Part model, mm, in its own coordinate system. A direction names the side the tool comes from. Give positions to 0.01 mm unless a question says otherwise; leave off trailing zeros. Write each loop counter-clockwise with the first axis right and the second up, starting at its lowest first coordinate (ties: lowest second). Pieces come first, ordered by that corner, then holes.
from build123d import *

# Parameters (mm, degrees)
SKETCH1_R           = 1
BOSS_EXTRUDE1_DEPTH = 15
SKETCH2_R           = 1
CUT_EXTRUDE1_DEPTH  = 105.560998943
FILLET1_R           = 0.35
SKETCH4_R           = 1
SKETCH4_R_2         = 0.75
BOSS_EXTRUDE2_DEPTH = 15


with BuildPart() as part:
    # Sketch1 → Boss-Extrude1 (new body)
    with BuildSketch(Plane.XY):
        with BuildLine():
            Line((-3.91822664, -0.5), (-11.924682731, -0.5))
            Line((-11.924682731, -0.5), (-11.924682731, -3.5))
            Line((-11.924682731, -3.5), (-5.417794754, -3.5))
            ThreePointArc((-5.417794754, -3.5), (-2.957602121, -5.731935947), (0.287025, -6.443610529))
            Line((0.287025, -6.443610529), (97.091971847, -2.131518769))
            ThreePointArc((97.091971847, -2.131518769), (97.728368045, -2.205906231), (98.308583108, -2.477722522))
            ThreePointArc((98.308583108, -2.477722522), (103, 0), (98.308583108, 2.477722522))
            ThreePointArc((98.308583108, 2.477722522), (97.728368045, 2.205906231), (97.091971847, 2.131518769))
            Line((97.091971847, 2.131518769), (0.287025, 6.443610529))
            ThreePointArc((0.287025, 6.443610529), (-1.950218056, 6.148101295), (-3.948733974, 5.1))
            Line((-3.948733974, 5.1), (-6.571238743, 5.1))
            Line((-6.571238743, 5.1), (-6.571238743, 3.5))
            Line((-6.571238743, 3.5), (-11.924682731, 3.5))
            Line((-11.924682731, 3.5), (-11.924682731, 0.5))
            Line((-11.924682731, 0.5), (-3.91822664, 0.5))
            ThreePointArc((-3.91822664, 0.5), (-3.242430239, 2.255913594), (-1.830983342, 3.5))
            Line((-1.830983342, 3.5), (1.830983342, 3.5))
            ThreePointArc((1.830983342, 3.5), (2.255913594, -3.242430239), (-3.91822664, -0.5))
        make_face()
        Polygon((88.963478068, 1.645749001), (94.011025285, 1.447599375), (91.58632649, -0.977099421), align=None, mode=Mode.SUBTRACT)
        with BuildLine():
            ThreePointArc((3.206155917, -5.012291316), (5.643134431, -1.88614257), (5.575683387, 2.077078421))
            Line((5.575683387, 2.077078421), (12.307755133, -4.654993325))
            Line((12.307755133, -4.654993325), (3.206155917, -5.012291316))
        make_face(mode=Mode.SUBTRACT)
        Polygon((29.468467153, -3.981321833), (13.440872209, -4.610510983), (21.769264256, 3.717881064), align=None, mode=Mode.SUBTRACT)
        Polygon((44.134225049, -3.405593798), (30.60158423, -3.93683949), (37.633527485, 3.095103765), align=None, mode=Mode.SUBTRACT)
        Polygon((56.667764123, -2.91356946), (45.267342125, -3.361111456), (51.191324122, 2.562870541), align=None, mode=Mode.SUBTRACT)
        Polygon((67.379082477, -2.493079343), (57.800881199, -2.869087118), (62.777985726, 2.108017409), align=None, mode=Mode.SUBTRACT)
        Polygon((76.533108343, -2.133723259), (68.512199553, -2.448597), (72.680090819, 1.719294266), align=None, mode=Mode.SUBTRACT)
        Polygon((84.356252684, -1.826613081), (77.666225419, -2.089240916), (81.142552969, 1.387086634), align=None, mode=Mode.SUBTRACT)
        Polygon((91.042009123, -1.564152904), (85.48936976, -1.782130738), (88.374678359, 1.10317786), align=None, mode=Mode.SUBTRACT)
        Polygon((96.755739716, -1.339851173), (92.175126199, -1.519670561), (94.555342652, 0.860545892), align=None, mode=Mode.SUBTRACT)
        with Locations((100, 0)):
            Circle(SKETCH1_R, mode=Mode.SUBTRACT)
        Polygon((21.224946889, 4.304934547), (12.8520725, -4.067939842), (3.794955626, 4.989177032), align=None, mode=Mode.SUBTRACT)
        Polygon((30.01278452, -3.39426835), (22.358063966, 4.260452205), (37.089210118, 3.682157248), align=None, mode=Mode.SUBTRACT)
        Polygon((44.678542416, -2.818540315), (38.222327195, 3.637674906), (50.647006755, 3.149924024), align=None, mode=Mode.SUBTRACT)
        Polygon((57.21208149, -2.326515977), (51.780123831, 3.105441681), (62.233668359, 2.695070892), align=None, mode=Mode.SUBTRACT)
        Polygon((67.923399844, -1.90602586), (63.366785435, 2.650588549), (72.135773452, 2.306347749), align=None, mode=Mode.SUBTRACT)
        Polygon((77.07742571, -1.546669776), (73.268890528, 2.261865406), (80.598235603, 1.974140117), align=None, mode=Mode.SUBTRACT)
        Polygon((84.900570051, -1.239559598), (81.731352679, 1.929657774), (87.830360992, 1.690231343), align=None, mode=Mode.SUBTRACT)
    extrude(amount=-BOSS_EXTRUDE1_DEPTH)

    # Sketch2 → Cut-Extrude1 (cut, through all)
    with BuildSketch(Plane(origin=(0, 3.5, 0), x_dir=(1, 0, 0), z_dir=(0, 1, 0))):
        with Locations(Location((-8.671238743, 11.25, 0), (0, 0, 270))):
            Circle(SKETCH2_R)
        with Locations(Location((-8.671238743, 3.75, 0), (0, 0, 270))):
            Circle(SKETCH2_R)
    extrude(amount=-CUT_EXTRUDE1_DEPTH, mode=Mode.SUBTRACT)

    # Fillet1
    fillet1_edges = [part.edges().sort_by_distance(p)[0] for p in [
        (92.175126199, -1.519670561, -7.5),
        (96.755739716, -1.339851173, -7.5),
        (94.555342652, 0.860545892, -7.5),
        (87.830360992, 1.690231343, -7.5),
        (81.731352679, 1.929657774, -7.5),
        (84.900570051, -1.239559598, -7.5),
        (88.963478068, 1.645749001, -7.5),
        (91.58632649, -0.977099421, -7.5),
        (94.011025285, 1.447599375, -7.5),
        (72.680090819, 1.719294266, -7.5),
        (68.512199553, -2.448597, -7.5),
        (76.533108343, -2.133723259, -7.5),
        (63.366785435, 2.650588549, -7.5),
        (67.923399844, -1.90602586, -7.5),
        (72.135773452, 2.306347749, -7.5),
        (57.800881199, -2.869087118, -7.5),
        (67.379082477, -2.493079343, -7.5),
        (62.777985726, 2.108017409, -7.5),
        (51.780123831, 3.105441681, -7.5),
        (57.21208149, -2.326515977, -7.5),
        (62.233668359, 2.695070892, -7.5),
        (45.267342125, -3.361111456, -7.5),
        (56.667764123, -2.91356946, -7.5),
        (51.191324122, 2.562870541, -7.5),
        (38.222327195, 3.637674906, -7.5),
        (44.678542416, -2.818540315, -7.5),
        (50.647006755, 3.149924024, -7.5),
        (30.60158423, -3.93683949, -7.5),
        (44.134225049, -3.405593798, -7.5),
        (37.633527485, 3.095103765, -7.5),
        (3.794955626, 4.989177032, -7.5),
        (12.8520725, -4.067939842, -7.5),
        (21.224946889, 4.304934547, -7.5),
        (13.440872209, -4.610510983, -7.5),
        (29.468467153, -3.981321833, -7.5),
        (21.769264256, 3.717881064, -7.5),
        (37.089210118, 3.682157248, -7.5),
        (22.358063966, 4.260452205, -7.5),
        (30.01278452, -3.39426835, -7.5),
        (73.268890528, 2.261865406, -7.5),
        (77.07742571, -1.546669776, -7.5),
        (80.598235603, 1.974140117, -7.5),
        (81.142552969, 1.387086634, -7.5),
        (77.666225419, -2.089240916, -7.5),
        (84.356252684, -1.826613081, -7.5),
        (91.042009123, -1.564152904, -7.5),
        (88.374678359, 1.10317786, -7.5),
        (85.48936976, -1.782130738, -7.5),
        (3.206155917, -5.012291316, -7.5),
        (12.307755133, -4.654993325, -7.5),
        (5.575683387, 2.077078421, -7.5),
        (-5.417794754, -3.5, -7.5),
        (-11.924682731, -3.5, -7.5),
        (-11.924682731, -0.5, -7.5),
        (-3.91822664, -0.5, -7.5),
        (1.830983342, 3.5, -7.5),
        (-1.830983342, 3.5, -7.5),
        (-3.91822664, 0.5, -7.5),
        (-11.924682731, 0.5, -7.5),
        (-11.924682731, 3.5, -7.5),
        (-6.571238743, 3.5, -7.5),
        (-6.571238743, 5.1, -7.5),
        (-3.948733974, 5.1, -7.5),
    ]]
    fillet(fillet1_edges, radius=FILLET1_R)

    # Sketch4 → Boss-Extrude2 (add)
    with BuildSketch(Plane.XY):
        with Locations((100, 0)):
            Circle(SKETCH4_R)
        with Locations((100, 0)):
            Circle(SKETCH4_R_2, mode=Mode.SUBTRACT)
    extrude(amount=-BOSS_EXTRUDE2_DEPTH)


solid = part.part
1) Saw through at B-B (z = -3.75). State how many separate pieces and enclosed holes the cut face has, and give its area (3 significant figures).
Check result:
separate pieces: 3
enclosed holes: 18
area: 433 mm2
2) Drill centre lines: L1, parallel to Y at x = 70, z = -13; L2, parallel to Y at x = 71.5, z = -8.5; L3, parallel to Y at x = 100, z = -9.5. Where is each one in solid material? Low to high.
Check result:
L1: y = -3.34 to -2.39, -0.96 to 0.17, 2.39 to 3.34
L2: y = -3.27 to -2.33, 0.54 to 1.67, 2.29 to 3.27
L3: y = -3 to -0.75, 0.75 to 3
3) Saw through at A-A (x = 17.5). Write the cut outline in (y, z), and give its area (3 significant figures).
Check result:
outline: (-5.68, -15) - (-4.45, -15) - (-4.45, 0) - (-5.68, 0) - close; (-0.55, -15) - (0.58, -15) - (0.58, 0) - (-0.55, 0) - close; (4.45, -15) - (5.68, -15) - (5.68, 0) - (4.45, 0) - close
area: 53.7 mm2
4) 3-axis set-ups, long thin cutter, end or side, ignore diameter. For faces 3 (the flat face through (26.43, 0.19, -7.4)), 4 (the flat face through (-9, 3.5, -7)), 5 (the flat face through (41, 0.5, -15)): which of +Z, -Z, +X, -X, +Y, -Y reach the whole face in a straight line?
Check result:
face 3: +Z, -Z
face 4: +Z, -Z, -X, +Y
face 5: -Z, +X, -X, +Y, -Y
5) Saw through at C-C (x = 54). Write the cut outline in (y, z).
Check result:
outline: (-4.05, -15) - (-3.02, -15) - (-3.02, 0) - (-4.05, 0) - close; (-0.25, -15) - (0.89, -15) - (0.89, 0) - (-0.25, 0) - close; (3.02, -15) - (4.05, -15) - (4.05, 0) - (3.02, 0) - close
6) Mould opens along X. For faces 1 (the flat face through (57, 2.9, -7.4)), 2 (the flat face through (41, 0.5, 0)) say: +X half, -X half, draft (parallel to the pull), parting line (faces both ways), or undercut.
Check result:
face 1: undercut
face 2: draft
7) Flat gauge pins, fed straight in: P1, Ø6, axis at x = 91.5, z = -10.5, coming from the +Y side; P2, Ø0.7, axis at y = 4.5, z = -9.5, coming from the -X side; P3, Ø2.5, axis at x = -8.67, z = -11.25, coming from the +Y side. Where does each tip first touch, or does it go through?
Check result:
P1: stops at y = 2.51
P2: stops at x = -6.57
P3: stops at y = 3.5
